```python
from build123d import *

# Parameters (mm, degrees)
F0_W     = 38
F0_H     = 18.5
F0_R     = 1.5
F0_W_2   = 10
F0_R_2   = 1.75
F1_DEPTH = 5
F2_W     = 25
F2_H     = 18.5
F3_DEPTH = 9.25
F5_DEPTH = 25


with BuildPart() as f1:
    # F0 (on Top) → F1 (new body)
    with BuildSketch(Plane.XY):
        Rectangle(F0_W, F0_H)
        with Locations((-16.65, 0)):
            Circle(F0_R, mode=Mode.SUBTRACT)
        with Locations((16.65, 0)):
            Circle(F0_R, mode=Mode.SUBTRACT)
        with Locations((24, 0)):
            Rectangle(F0_W_2, F0_H)
        with Locations((25, 0)):
            Circle(F0_R_2, mode=Mode.SUBTRACT)
        with Locations((-24, 0)):
            Rectangle(F0_W_2, F0_H)
        with Locations((-25, 0)):
            Circle(F0_R_2, mode=Mode.SUBTRACT)
    extrude(amount=F1_DEPTH)

    # F2 (on face) → F3 (join)
    with BuildSketch(Plane.XY.offset(5)):
        Rectangle(F2_W, F2_H)
    extrude(amount=F3_DEPTH)

    # F4 (on face) → F5 (cut)
    with BuildSketch(Plane(origin=(-12.5, 0, 0), x_dir=(0, -1, 0), z_dir=(-1, 0, 0))):
        with BuildLine():
            ThreePointArc((-9.25, 5), (-6.540737726, 11.540737726), (0, 14.25))
            Line((0, 14.25), (-9.25, 14.25))
            Line((-9.25, 14.25), (-9.25, 5))
        make_face()
        with BuildLine():
            ThreePointArc((0, 14.25), (6.540737726, 11.540737726), (9.25, 5))
            Line((9.25, 5), (9.25, 14.25))
            Line((9.25, 14.25), (0, 14.25))
        make_face()
    extrude(amount=-F5_DEPTH, mode=Mode.SUBTRACT)


solid = f1.part
```
Model file for the job. Use its own axes, mm. A direction names the side the tool comes from. Give positions to 0.01 mm unless a question says otherwise; leave off trailing zeros. Loops run counter-clockwise (first coordinate to the right, second up) from the corner with the lowest first, then second, coordinate; pieces in that order, holes last. Notation, with made-up numbers: (41.5, -11.75) - (73.5, -11.75) arc R26 cw to (73.5, 4.25) - close; hole circle Ø11 at (-15, 68). An arc over 180 degrees is marked (long way). One line per item, written item: value. Start each with the question number.
1. Probe L1, parallel to Y at x = -25, z = 3.05; L2, parallel to Y at x = 16.65, z = 2.9; L3, parallel to X at y = 1, z = 4.25. List the from-to ranges inside material, lowest first. Write a range as from..to.
2. Slice it at C-C (y = 5.5). List the corners of the cut face in (x, z).
3. Slice it at A-A (x = -16.65). List the corners of the cut face in (y, z), plus the area to 3 significant figures.
4. Which spindle directions (+Z, -Z, +X, -X, +Y, -Y) get a long thin tool onto all of the face, cutting with end or side? Do faces 1 (the cylindrical face through (-18.15, 0.07, 2.46)), 2 (the flat face through (-21, 0, 5)), 3 (the flat face through (12.5, 0, 9)). Say none if no direction does.
5. Slice it at D-D (x = 6). List the corners of the cut face in (y, z).
6. Pin check, flat tips, straight feed: pin 1 (4 mm diameter, centred on x = 19.5, y = 6, fed in from -Z); pin 2 (2.5 mm diameter, centred on x = 16.65, y = 0, fed in from +Z); pin 3 (8 mm diameter, centred on x = 15, z = 11.5, fed in from +Y); pin 4 (3.5 mm diameter, centred on x = -16.65, y = 0, fed in from +Z). Stop position of each tip, or through.
7. Slice it at B-B (z = 2.75). List the corners of the cut face in (x, y).
8. Pull direction Y, two halves, no side cores. Call faces 4 (the cylindrical face through (18.08, 0.45, 2.46)), 5 (the flat face through (0, -9.25, 2)), 6 (the flat face through (-29, 0, 2)): pulls with the +Y half, pulls with the -Y half, needs draft (parallel to the pull), parting line crosses it, or undercut.
Solution:
1. L1: y = -9.25..-1.75, 1.75..9.25
1. L2: y = -9.25..-1.5, 1.5..9.25
1. L3: x = -29..-26.44, -23.56..-17.77, -15.53..15.53, 17.77..23.56, 26.44..29
2. outline: (-29, 0) - (29, 0) - (29, 5) - (12.5, 5) - (12.5, 12.44) - (-12.5, 12.44) - (-12.5, 5) - (-29, 5) - close
3. outline: (-9.25, 0) - (-1.5, 0) - (-1.5, 5) - (-9.25, 5) - close; (1.5, 0) - (9.25, 0) - (9.25, 5) - (1.5, 5) - close
3. area: 77.5 mm^2
4. face 1: +Z, -Z
4. face 2: +Z, -X, +Y, -Y
4. face 3: +Z, +X, +Y, -Y
5. outline: (-9.25, 0) - (9.25, 0) - (9.25, 5) arc R9.25 ccw to (-9.25, 5) - close
6. pin 1: stops at z = 0
6. pin 2: passes through
6. pin 3: stops at y = 8.61
6. pin 4: stops at z = 5
7. outline: (-29, -9.25) - (29, -9.25) - (29, 9.25) - (-29, 9.25) - close; hole circle Ø3.5 at (-25, 0); hole circle Ø3 at (-16.65, 0); hole circle Ø3 at (16.65, 0); hole circle Ø3.5 at (25, 0)
8. face 4: undercut
8. face 5: pulls with the -Y half
8. face 6: needs draft
